Autodesk Inventor part; units mm, degrees
ref_plane "YZ Plane" through (0, 0, 0) normal (1, 0, 0) x (0, 1, 0)
ref_plane "XZ Plane" through (0, 0, 0) normal (0, 1, 0) x (-1, 0, 0)
ref_plane "XY Plane" through (0, 0, 0) normal (0, 0, 1) x (1, 0, 0)
sketch "Sketch2" plane through (0, 0, 0) normal (0, 0, 1) x (1, 0, 0)
  circle A0 centre (0, 0) radius 152.4
  circle A1 centre (0, 0) radius 137.16
  circle A2 centre (0, 106.68) radius 11.43
  circle A3 centre (-53.34, 92.3876) radius 11.43
  circle A4 centre (-92.3876, 53.34) radius 11.43
  circle A5 centre (-106.68, 0) radius 11.43
  circle A6 centre (-92.3876, -53.34) radius 11.43
  circle A7 centre (-53.34, -92.3876) radius 11.43
  circle A8 centre (0, -106.68) radius 11.43
  circle A9 centre (53.34, -92.3876) radius 11.43
  circle A10 centre (92.3876, -53.34) radius 11.43
  circle A11 centre (106.68, 0) radius 11.43
  circle A12 centre (92.3876, 53.34) radius 11.43
  circle A13 centre (53.34, 92.3876) radius 11.43
  dimension "d0" = 304.8
  dimension "d1" = 274.32
  dimension "d2" = 22.86
  dimension "d5" = 360
extrude "Extrusion1" add sketch "Sketch2" against normal blind 27.432 contours A1
extrude "Extrusion2" add sketch "Sketch2" against normal blind 18.288 contours A0
sketch "Sketch3" plane through (0, 0, -27.432) normal (0, 0, -1) x (-1, 0, 0)
  circle A0 centre (0, 0) radius 83.82
  dimension "d11" = 167.64
extrude "Extrusion3" add sketch "Sketch3" along normal blind 914.4
sketch "Sketch4" plane through (0, 0, -941.832) normal (0, 0, -1) x (-1, 0, 0)
  circle A0 centre (0, 0) radius 60.96
  dimension "d14" = 121.92
extrude "Extrusion4" cut sketch "Sketch4" against normal blind 1524
mirror "Mirror2" about plane through (0, 0, 0) normal (0, 0, 1) of "Extrusion2", "Extrusion1", "Extrusion3", "Extrusion4"
properties part number "fuel_pipeline"
The model under review builds one solid part; all positions refer to its coordinate system, in mm. A direction names the side the tool comes from. Give positions to 0.01 mm unless a question says otherwise; leave off trailing zeros. Loops run counter-clockwise (first coordinate to the right, second up) from the corner with the lowest first, then second, coordinate; pieces in that order, holes last. Notation, with made-up numbers: (54.5, 56.5) -> (68.5, 56.5) arc R22 ccw to (68.5, 65.5) -> close; hole circle Ø8 at (-17.75, 85). An arc over 180 degrees is marked (long way). Answer as a JSON object with one key per item and string values. Group by question number.
Q1. Wall thickness on line 1 along Y through (x, z) = (0, -14); line 2 along Y through (x, z) = (53.34, -1); line 3 along X through (y, z) = (53, -7): over which ranges is each line inside the solid? List them lowest first.
Q2. Tool access review of faces 1 (the flat face through (-90, 2, 27.432)), 2 (the flat face through (-6, -62, -941.832)), 3 (the cylindrical face through (73.74, 115.65, -22.8)): name each direction out of +Z, -Z, +X, -X, +Y, -Y from which nothing blocks a thin tool from reaching the whole face with its end or side.
Q3. Insertion check: pin 1 (6 mm diameter, centred on x = -50.5, z = -695.5, fed in from -Y); pin 2 (5 mm diameter, centred on x = -10, y = 84.5, fed in from +Z); pin 3 (2 mm diameter, centred on x = 73.5, y = 45.5, fed in from -Z); pin 4 (4 mm diameter, centred on x = 75, z = 168, fed in from -Y). Each pin has a flat end and moves straight along its axis. Give the tip position at first contact, or say it passes through.
Q4. Draft analysis for pull direction Y (two halves, no side actions). For faces 4 (the cylindrical face through (13.21, -59.51, -13.19)), 5 (the cylindrical face through (10.912, -83.107, -478.231)), 6 (the flat face through (90, 2, -27.432)), state which applies: pulls with the +Y half, pulls with the -Y half, needs draft (parallel to the pull), parting line crosses it, or undercut.
Q5. Take a section at A-A (z = -418). Write out the cut boundary in (x, y), plus the area to 3 significant figures.
Answer below:
{
 "1": {"line 1": "y = -152.4 to -118.11, -95.25 to -60.96, 60.96 to 95.25, 118.11 to 152.4", "line 2": "y = -142.76 to -103.82, -80.96 to -29.51, 29.51 to 80.96, 103.82 to 142.76", "line 3": "x = -142.89 to -103.81, -80.96 to -30.12, 30.12 to 80.96, 103.81 to 142.89"},
 "2": {"face 1": "+Z", "face 2": "-Z, +X, -X, +Y, -Y", "face 3": "-Z"},
 "3": {"pin 1": "stops at y = -69.06", "pin 2": "stops at z = 941.83", "pin 3": "stops at z = -27.43", "pin 4": "stops at y = -41.19"},
 "4": {"face 4": "undercut", "face 5": "parting line crosses it", "face 6": "needs draft"},
 "5": {"outline": "circle Ø167.64 at (0, 0); hole circle Ø121.92 at (0, 0)", "area": "10,400 mm2"}
}
